Source: three-view drawing plus pictorial views. Frame: mm from the lowest corner of the part. Coordinates: 2 decimals unless noted, no trailing zeros. Write each loop counter-clockwise with the first axis right and the second up, starting at its lowest first coordinate (ties: lowest second). Pieces come first, ordered by that corner, then holes. Notation, with made-up numbers: (-30, 39.5) -> (25, 39.5) arc R19 ccw to (25, 51.5) -> close; hole circle Ø10 at (77, 21). An arc over 180 degrees is marked (long way). Write item = value, one per line.
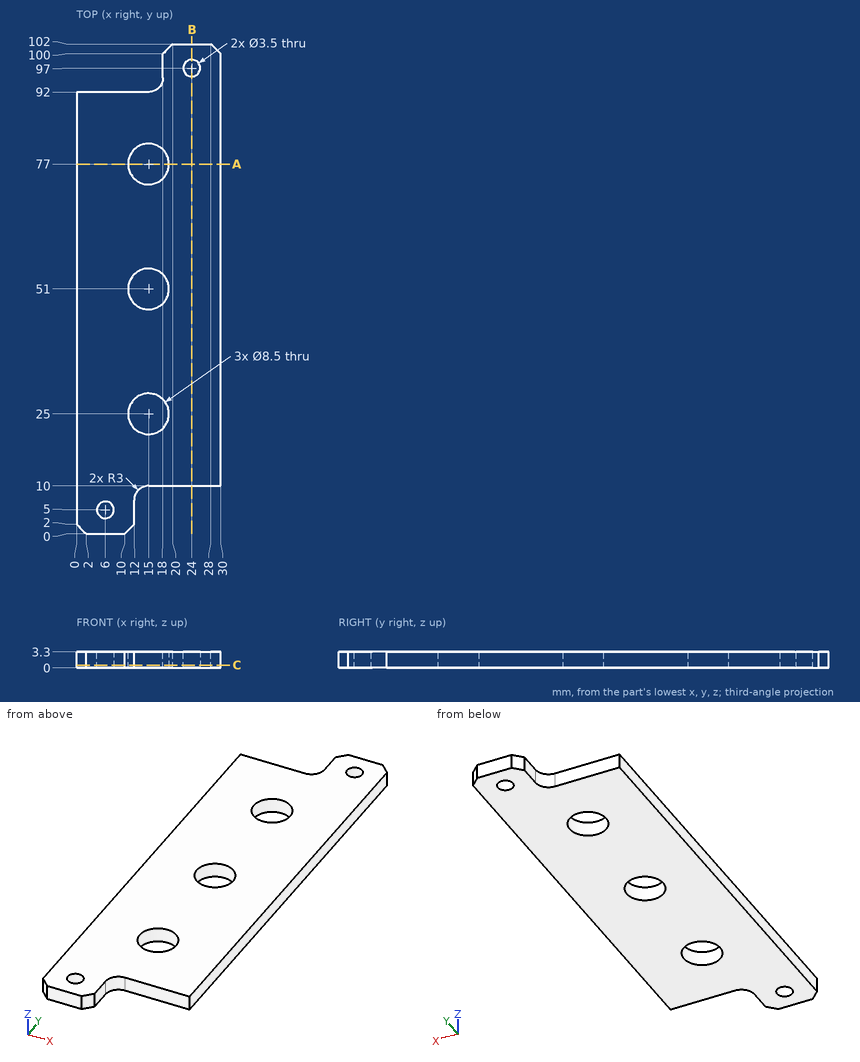
1) Material intervals for probe 1 along Y at (x, z) = (15.25, 1); probe 2 along Y at (x, z) = (6, 1); probe 3 along Y at (x, z) = (11.75, 0.5), sorted ascending. Write a range as [from, to].
Answer block:
probe_1 = [10, 20.76], [29.24, 46.76], [55.24, 72.76], [81.24, 92.01]
probe_2 = [0, 3.25], [6.75, 92]
probe_3 = [1.75, 22.26], [27.74, 48.26], [53.74, 74.26], [79.74, 92]
2) Cut plane C-C, the plane z = 0.55. Output: boundary loops of the cut face in (x, y), and give its area (3 significant figures).
Answer block:
outline = (0, 2) -> (2, 0) -> (10, 0) -> (12, 2) -> (12, 7) arc R3 cw to (15, 10) -> (30, 10) -> (30, 100) -> (28, 102) -> (20, 102) -> (18, 100) -> (18, 95) arc R3 cw to (15, 92) -> (0, 92) -> close; hole circle Ø3.5 at (6, 5); hole circle Ø8.5 at (15, 25); hole circle Ø8.5 at (15, 51); hole circle Ø8.5 at (15, 77); hole circle Ø3.5 at (24, 97)
area = 2,510 mm2
3) First-contact query: pin 1 Ø8 at (x, y) = (26.5, 30) entering from -Z; pin 2 Ø1 at (y, z) = (5.5, 2.5) entering from +X. Flat tips, straight axial feed; report the tip coordinate or a pass-through.
Answer block:
pin_1 = 0
pin_2 = 12
4) Cut plane B-B, the plane x = 24. Output: boundary loops of the cut face in (y, z), and give its area (3 significant figures).
Answer block:
outline = (10, 0) -> (95.25, 0) -> (95.25, 3.3) -> (10, 3.3) -> close; (98.75, 0) -> (102, 0) -> (102, 3.3) -> (98.75, 3.3) -> close
area = 292 mm2
5) Cut plane A-A, the plane y = 77. Output: boundary loops of the cut face in (x, z), and give its area (4 significant figures).
Answer block:
outline = (0, 0) -> (10.75, 0) -> (10.75, 3.3) -> (0, 3.3) -> close; (19.25, 0) -> (30, 0) -> (30, 3.3) -> (19.25, 3.3) -> close
area = 70.95 mm2
